The model under review builds one solid part; all positions refer to its coordinate system, in mm. Face numbers are marked on the shaded views. Give positions to 0.01 mm unless a question says otherwise; leave off trailing zeros. Order: outer loops, then holes, each group sorted by start corner. A loop starts at its lowest first (then second) coordinate and runs counter-clockwise, first axis right, second up. Notation, with made-up numbers: (-26.5, 21.5) - (23.5, 21.5) arc R7 cw to (23.5, 28.5) - close; hole circle Ø4 at (-35, -9). An arc over 180 degrees is marked (long way). Use CSV: the item, a comma, the result in double quotes. Start each with the question number.
1. Draft analysis for pull direction Z (two halves, no side actions). For the marked faces 1, 2 and 3, state which applies: released by +Z, released by -Z, zero draft, split by the parting line, or undercut.
2. To check wall thickness, follow line 1 (Y direction, x = 2.5, z = 3.75); line 2 (Y direction, x = -1.75, z = -2.75); line 3 (X direction, y = 17.7, z = 0). State the ranges of each line that lie inside material, in increasing order. Write a range as [from, to].
3. Take a section at C-C, the plane x = 0. State the section outline as (y, z) points, then the cut area to 3 significant figures.
4. For pin 1 (1.5 mm diameter, centred on y = 15, z = 4, fed in from -X); pin 2 (3 mm diameter, centred on x = 0, z = -1, fed in from -Y); pin 3 (4.5 mm diameter, centred on x = 0, z = 0, fed in from +Y), all flat-tipped, find the tip position at first contact; note any pin that passes through.
5. Take a section at B-B, the plane y = -0.5. State the section outline as (x, z) points (1 decimal).
6. Take a section at D-D, the plane y = 13.5. State the section outline as (x, z) points, then the cut area to 3 significant figures.
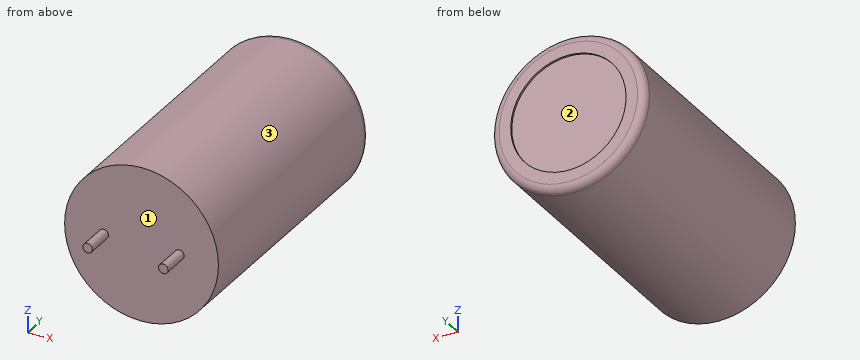
```python
from build123d import *

# Parameters (mm, degrees)
SKETCH1_R           = 5.08
BOSS_EXTRUDE1_DEPTH = 17.78
SKETCH2_R           = 0.3175
BOSS_EXTRUDE2_DEPTH = 1.905
SKETCH3_R           = 3.81
CUT_EXTRUDE1_DEPTH  = 0.127
FILLET1_R           = 0.508


with BuildPart() as part:
    # Sketch1 → Boss-Extrude1 (new body)
    with BuildSketch(Plane(origin=(0, 0, 0), x_dir=(1, 0, 0), z_dir=(0, 1, 0))):
        with Locations(Location((0, 0, 0), (0, 0, 270))):
            Circle(SKETCH1_R)
    extrude(amount=BOSS_EXTRUDE1_DEPTH)

    # Sketch2 → Boss-Extrude2 (add)
    with BuildSketch(Plane.XZ):
        with Locations(Location((-2.5, 0, 0), (0, 0, 90))):
            Circle(SKETCH2_R)
        with Locations(Location((2.5, 0, 0), (0, 0, 90))):
            Circle(SKETCH2_R)
    extrude(amount=BOSS_EXTRUDE2_DEPTH)

    # Sketch3 → Cut-Extrude1 (cut)
    with BuildSketch(Plane(origin=(0, 17.78, 0), x_dir=(1, 0, 0), z_dir=(0, 1, 0))):
        with Locations(Location((0, 0, 0), (0, 0, 270))):
            Circle(SKETCH3_R)
    extrude(amount=-CUT_EXTRUDE1_DEPTH, mode=Mode.SUBTRACT)

    # Fillet1
    fillet1_edges = [part.edges().sort_by_distance(p)[0] for p in [
        (0, 17.78, -5.08),
    ]]
    fillet(fillet1_edges, radius=FILLET1_R)


solid = part.part
```
Determined:
1,face 1,"zero draft"
1,face 2,"undercut"
1,face 3,"split by the parting line"
2,line 1,"y = [0, 17.78]"
2,line 2,"y = [0, 17.65]"
2,line 3,"x = [-4.85, -3.81], [3.81, 4.85]"
3,outline,"(0, -5.08) - (17.27, -5.08) arc R0.51 ccw to (17.78, -4.57) - (17.78, -3.81) - (17.65, -3.81) - (17.65, 3.81) - (17.78, 3.81) - (17.78, 4.57) arc R0.51 ccw to (17.27, 5.08) - (0, 5.08) - close"
3,area,"180 mm²"
4,pin 1,"stops at x = -3.9"
4,pin 2,"stops at y = 0"
4,pin 3,"stops at y = 17.65"
5,outline,"circle Ø0.6 at (-2.5, 0); circle Ø0.6 at (2.5, 0)"
6,outline,"circle Ø10.16 at (0, 0)"
6,area,"81.1 mm²"
